Could you check a few things on this model? Use its own coordinates, in mm. Coordinates: 2 decimals unless noted, no trailing zeros. Write each loop counter-clockwise with the first axis right and the second up, starting at its lowest first coordinate (ties: lowest second). Pieces come first, ordered by that corner, then holes.
Item 1: I want a section at A-A on x = 0. Please give me the cut outline in (y, z), then the cut area to 3 significant figures.
Item 2: If I drill on probe 1 along Y at (x, z) = (0, 23); probe 2 along Z at (x, y) = (-5.5, 0.75); probe 3 along X at (y, z) = (2.5, 21.5), over which ranges is the centre line in solid material (lowest first)?
Item 3: For P1, Ø4, axis at x = 3, z = 22.5, coming from the +Y side; P2, Ø3, axis at x = -1.5, y = -1, coming from the -Z side; P3, Ø1, axis at y = -3, z = 33, coming from the -X side; P4, Ø4, axis at x = -2.5, z = 29, coming from the -Y side, each with a flat end and sliding along its axis, tell me the tip position at first contact or that it passes through.
Item 4: I want a section at C-C on z = 23.5. Please give me the cut outline in (x, y), then the cut area to 3 significant figures.
Item 5: Thinking about a two-plate mould opening in Y: for faces 1 (the cylindrical face through (-6, 0, 20)), 2 (the cylindrical face through (3.233, -1.341, 19.72)), 3 (the flat face through (4, 0, 0)), which applies, +Y half, -Y half, draft (parallel to the pull), parting line (faces both ways), or undercut?
from build123d import *

# Parameters (mm, degrees)
SKETCH1_R           = 6
SKETCH1_R_2         = 3.5
BOSS_EXTRUDE1_DEPTH = 40
FILLET1_R           = 0.5
FILLET2_R           = 0.5


with BuildPart() as part:
    # Sketch1 → Boss-Extrude1 (new body)
    with BuildSketch(Plane.XY):
        Circle(SKETCH1_R)
        Circle(SKETCH1_R_2, mode=Mode.SUBTRACT)
    extrude(amount=BOSS_EXTRUDE1_DEPTH)

    # Fillet1
    fillet1_edges = [part.edges().sort_by_distance(p)[0] for p in [
        (-6, 0, 40),
    ]]
    fillet(fillet1_edges, radius=FILLET1_R)

    # Fillet2
    fillet2_edges = [part.edges().sort_by_distance(p)[0] for p in [
        (-6, 0, 0),
    ]]
    fillet(fillet2_edges, radius=FILLET2_R)


solid = part.part
Response values:
1. outline: (-6, 0.5) arc R0.5 ccw to (-5.5, 0) - (-3.5, 0) - (-3.5, 40) - (-5.5, 40) arc R0.5 ccw to (-6, 39.5) - close; (3.5, 0) - (5.5, 0) arc R0.5 ccw to (6, 0.5) - (6, 39.5) arc R0.5 ccw to (5.5, 40) - (3.5, 40) - close
1. area: 200 mm2
2. probe 1: y = -6 to -3.5, 3.5 to 6
2. probe 2: z = 0 to 40
2. probe 3: x = -5.45 to -2.45, 2.45 to 5.45
3. P1: stops at y = 5.92
3. P2: passes through
3. P3: stops at x = -5.45
3. P4: stops at y = -5.98
4. outline: circle Ø12 at (0, 0); hole circle Ø7 at (0, 0)
4. area: 74.6 mm2
5. face 1: parting line
5. face 2: undercut
5. face 3: draft
